Job drawing, mm, ordinate dimensions from the low corner. One solid piece. A direction names the side the tool comes from. Round coordinates to 2 decimals unless told otherwise and drop trailing zeros. Loops run counter-clockwise (first coordinate to the right, second up) from the corner with the lowest first, then second, coordinate; pieces in that order, holes last.
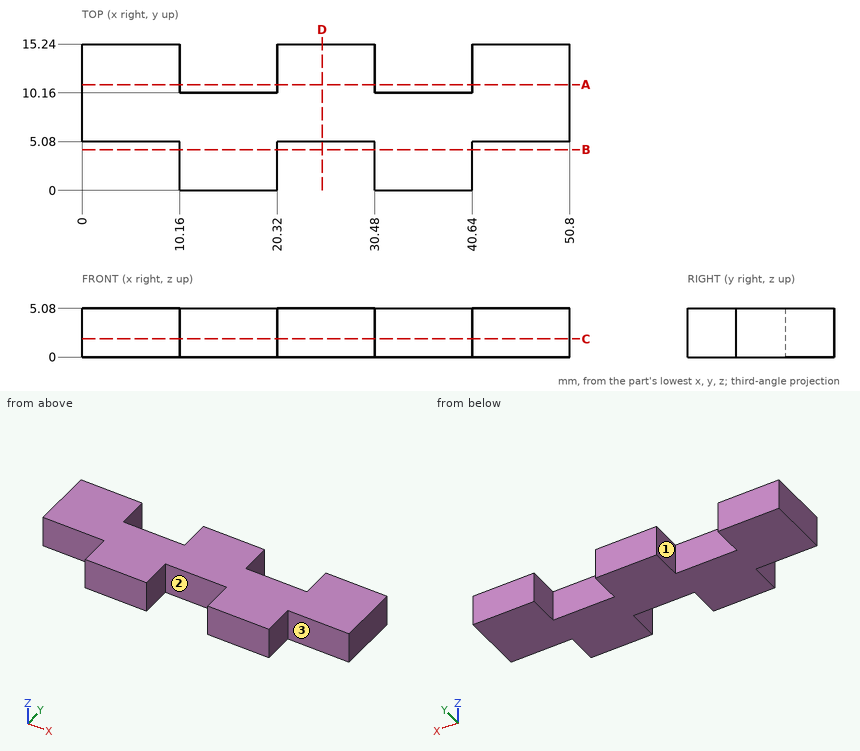
Item 1: 3-axis set-ups, long thin cutter, end or side, ignore diameter. For the marked faces 1, 2 and 3: which of +Z, -Z, +X, -X, +Y, -Y reach the whole face in a straight line?
Answers follow:
face 1: +Z, -Z, +Y
face 2: +Z, -Z, -Y
face 3: +Z, -Z, +X, -Y
Item 2: Probe line 1 (X direction, y = 13.5, z = 3.6); line 2 (X direction, y = 4.5, z = 3.7); line 3 (Y direction, x = 13, z = 1.2). List the from-to ranges inside material, lowest first.
Answers follow:
line 1: x = 0 to 10.16, 20.32 to 30.48, 40.64 to 50.8
line 2: x = 10.16 to 20.32, 30.48 to 40.64
line 3: y = 0 to 10.16
Item 3: Flat gauge pins, fed straight in: P1, Ø1.5, axis at y = 1.5, z = 3.5, coming from the -X side; P2, Ø2.5, axis at y = 13.5, z = 1.5, coming from the -X side; P3, Ø2.5, axis at x = 4.5, z = 1.5, coming from the -Y side; P4, Ø1.5, axis at x = 34.5, z = 2, coming from the +Y side. Where does each tip first touch, or does it go through?
Answers follow:
P1: stops at x = 10.16
P2: stops at x = 0
P3: stops at y = 5.08
P4: stops at y = 10.16
Item 4: Cut at D-D, the plane x = 25. Give the cut face in (y, z), plus the area to 3 significant figures.
Answers follow:
outline: (5.08, 0) - (15.24, 0) - (15.24, 5.08) - (5.08, 5.08) - close
area: 51.6 mm2
Item 5: Cut at C-C, the plane z = 1.9. Give the cut face in (x, y).
Answers follow:
outline: (0, 5.08) - (10.16, 5.08) - (10.16, 0) - (20.32, 0) - (20.32, 5.08) - (30.48, 5.08) - (30.48, 0) - (40.64, 0) - (40.64, 5.08) - (50.8, 5.08) - (50.8, 15.24) - (40.64, 15.24) - (40.64, 10.16) - (30.48, 10.16) - (30.48, 15.24) - (20.32, 15.24) - (20.32, 10.16) - (10.16, 10.16) - (10.16, 15.24) - (0, 15.24) - close
Item 6: Cut at B-B, the plane y = 4.25. Give the cut face in (x, z).
Answers follow:
outline: (10.16, 0) - (20.32, 0) - (20.32, 5.08) - (10.16, 5.08) - close; (30.48, 0) - (40.64, 0) - (40.64, 5.08) - (30.48, 5.08) - close
Item 7: Cut at A-A, the plane y = 11. Give the cut face in (x, z), plus the area to 3 significant figures.
Answers follow:
outline: (0, 0) - (10.16, 0) - (10.16, 5.08) - (0, 5.08) - close; (20.32, 0) - (30.48, 0) - (30.48, 5.08) - (20.32, 5.08) - close; (40.64, 0) - (50.8, 0) - (50.8, 5.08) - (40.64, 5.08) - close
area: 155 mm2
